Here's how the part is built. I have some questions about the finished solid (model axes, mm). A direction names the side the tool comes from. Coordinates: 2 decimals unless noted, no trailing zeros. Write each loop counter-clockwise with the first axis right and the second up, starting at its lowest first coordinate (ties: lowest second). Pieces come first, ordered by that corner, then holes.
Item 1: If we section it at B-B (x = 14.5): Count the separate pieces of the cut face and the enclosed holes in it, then the cut area to 3 significant figures.
Item 2: If we section it at A-A (y = -12): Please give me the cut outline in (x, z).
Item 3: If I drill on line 1 (Y direction, x = -15.5, z = 0); line 2 (X direction, y = -124.5, z = -4.5); line 3 (Y direction, x = 11.5, z = -14.5), over which ranges is the centre line in solid material (lowest first)?
Item 4: We'd pull the mould along Y, two halves only. Please class faces 1 (the face through (19.376, -73.95, 1.684)), 2 (the face through (0, 45, 0)), 3 (the face through (-2, 0, 8)): +Y half, -Y half, draft (parallel to the pull), parting line (faces both ways), or undercut.
Item 5: For faces 4 (the face through (-19.58, -73.95, 1.86)), 5 (the face through (18, -74, 7.995)), 6 (the face through (8.299, -73.95, -14.392)), 7 (the face through (2.09, 30.94, -9.39)), 8 (the face through (-4.133, -73.95, 16.16)), which set-ups out of +Z, -Z, +X, -X, +Y, -Y let a thin tool reach every point of the face, with its end or its side?
Item 6: I'm going to push flat-ended pins straight in: pin 1 Ø5 at (x, y) = (12.5, -99) entering from -Z; pin 2 Ø12 at (y, z) = (-35, 13) entering from +X; pin 3 Ø1 at (y, z) = (-18.5, 24.5) entering from -X. Where does each tip first touch, or does it pass through?
Item 7: If we section it at C-C (y = 22): Please give me the cut outline in (x, z), then the cut area to 3 significant figures.
from build123d import *

# Parameters (mm, degrees)
F1_DEPTH  = 150
F2_R      = 7.994771935
F3_DEPTH  = 30
F3_FACE_R = 7.994771935
F4_DEPTH  = 15
F4_TAPER  = -60


with BuildPart() as f1:
    # F0 (on Front) → F1 (new body)
    with BuildSketch(Plane.XZ):
        Polygon((8.3843320608, 7.994771935), (0, 24.09890946), (-8.3843320608, 7.994771935), (-26.7688590564, 7.994771935), (-12.1869118884, -4.4532320462), (-16.8345868587, -18.2800656185), (0, -10.6114018708), (16.8345868587, -18.2800656185), (12.1869118884, -4.4532320462), (26.7688590564, 7.994771935), align=None)
    extrude(amount=F1_DEPTH)

    # F2 (on face) → F3 (join)
    with BuildSketch(Plane(origin=(0, 0, 0), x_dir=(-1, 0, 0), z_dir=(0, 1, 0))):
        Circle(F2_R)
    extrude(amount=F3_DEPTH)

    # F3_face (on face) → F4 (join)
    with BuildSketch(Plane(origin=(0, 30, 0), x_dir=(-1, 0, 0), z_dir=(0, 1, 0))):
        Circle(F3_FACE_R)
    extrude(amount=F4_DEPTH, taper=F4_TAPER)


solid = f1.part
Answer list:
1. separate pieces: 3
1. enclosed holes: 0
1. area: 2,870 mm2
2. outline: (-26.77, 7.99) - (-12.19, -4.45) - (-16.83, -18.28) - (0, -10.61) - (16.83, -18.28) - (12.19, -4.45) - (26.77, 7.99) - (8.38, 7.99) - (0, 24.1) - (-8.38, 7.99) - close
3. line 1: y = -150 to 0, 34.33 to 45
3. line 2: x = -12.2 to 12.2
3. line 3: y = -150 to 0, 36.07 to 45
4. face 1: draft
4. face 2: +Y half
4. face 3: undercut
5. face 4: -X, -Y
5. face 5: +Z, +X, -Y
5. face 6: -Z, -Y
5. face 7: none
5. face 8: +Z, -X, -Y
6. pin 1: stops at z = -17.44
6. pin 2: stops at x = 26.77
6. pin 3: stops at x = -0.05
7. outline: circle Ø15.99 at (0, 0)
7. area: 201 mm2
